Part model, mm, in its own coordinate system. A direction names the side the tool comes from. Round coordinates to 2 decimals unless told otherwise and drop trailing zeros. Loops run counter-clockwise (first coordinate to the right, second up) from the corner with the lowest first, then second, coordinate; pieces in that order, holes last. Notation, with made-up numbers: (12, 43) -> (71, 43) arc R8 ccw to (71, 52) -> close; hole circle Ø2 at (49, 22.25). An arc over 180 degrees is marked (long way). Answer as CSV lines item,"result".
Solid Edge part; units mm, degrees
sketch "Sketch1" plane through (0, 0, 0) normal (0, -1, 0) x (1, 0, 0)
  line L0 (0, 0) -> (22.5, 0)
  line L1 (22.5, 0) -> (22.5, 5)
  line L2 (22.5, 5) -> (-5, 5)
  line L3 (-5, 5) -> (-5, -41)
  line L4 (-5, -41) -> (22.5, -41)
  line L5 (22.5, -41) -> (22.5, -36)
  line L6 (22.5, -36) -> (0, -36)
  line L7 (0, -36) -> (0, 0)
  dimension "D1" = 22.5
  dimension "D2" = 22.5
  dimension "D3" = 22.5
extrude "Protrusion1" add sketch "Sketch1" along normal mid plane 25
sketch "Sketch2" plane through (7.5, 0, 5) normal (0, 0, 1) x (0, 1, 0)
  line L0 (-12.5, 0) -> (-5, -15)
  line L1 (-5, -15) -> (5, -15)
  line L2 (5, -15) -> (12.5, 0)
  line L3 (12.5, 0) -> (12.5, -17.5)
  line L4 (12.5, -17.5) -> (-12.5, -17.5)
  line L5 (-12.5, -17.5) -> (-12.5, 0)
  dimension "D1" = 12.5
  dimension "D2" = 5
extrude "Cutout1" cut sketch "Sketch2" against normal through all
fillet "Round_2" radius 7.5 4 edges at (22.5, -5, 2.5) (22.5, 5, 2.5) (22.5, -5, -38.5) (22.5, 5, -38.5)
hole "Hole_2" at (16, 0, 5) direction (0, 0, -1) diameter 4.5 end through all start chamfer 0.4 start chamfer angle 45 end chamfer 0.4 end chamfer angle 45
hole "Hole_3" at (16, 0, 5) direction (0, 0, -1) diameter 7.2 end up to next
sketch "Sketch3" plane through (7.5, 0, 5) normal (0, 0, 1) x (0, 1, 0)
  line L0 (-3.6, -8.5) -> (3.6, -8.5)
  line L1 (3.6, -8.5) -> (2.4993, 11.5)
  line L2 (2.4993, 11.5) -> (-2.4993, 11.5)
  line L3 (-2.4993, 11.5) -> (-3.6, -8.5)
extrude "ExtrudedCutout_2" cut sketch "Sketch3" against normal blind 2.5
hole "Hole1" at (0, 0, -25.5) direction (-1, 0, 0) diameter 4.5 depth 30 tip angle 118 start chamfer 0.4 start chamfer angle 45 end chamfer 0.4 end chamfer angle 45
hole "Hole2" at (0, 0, -10.5) direction (-1, 0, 0) diameter 4.5 depth 30 tip angle 118 start chamfer 0.4 start chamfer angle 45 end chamfer 0.4 end chamfer angle 45
hole "Hole_8" at (0, -7.5, -18) direction (-1, 0, 0) diameter 3.7 depth 30 tip angle 118 start chamfer 0.6 start chamfer angle 45 end chamfer 0.6 end chamfer angle 45
hole "Hole3" at (0, 7.5, -18) direction (-1, 0, 0) diameter 3.7 depth 30 tip angle 118 start chamfer 0.6 start chamfer angle 45 end chamfer 0.6 end chamfer angle 45
properties material "Polypropylene, general purpose"
Q1. Drop flat-ended pins along their axis: P1, Ø7, axis at x = 16, y = 0, coming from the +Z side; P2, Ø2, axis at y = -8.5, z = 0, coming from the +X side; P3, Ø2, axis at x = 6.5, y = 1.5, coming from the +Z side. Give the stop position or say it passes through.
Geometry results:
P1,"z = -36"
P2,"x = 17.5"
P3,"z = 2.5"
Q2. Saw through at D-D, the plane x = 14.25. Give the number of separate pieces and of enclosed holes in the cut face, then the cut area to 3 significant figures.
Geometry results:
separate pieces,"4"
enclosed holes,"0"
area,"135 mm2"
Q3. Saw through at C-C, the plane x = 3.5. Write the cut outline in (y, z).
Geometry results:
outline,"(-12.5, -41) -> (12.5, -41) -> (12.5, -36) -> (-12.5, -36) -> close; (-12.5, 0) -> (12.5, 0) -> (12.5, 5) -> (2.91, 5) -> (2.91, 2.5) -> (-2.91, 2.5) -> (-2.91, 5) -> (-12.5, 5) -> close"
Q4. Two-plate mould, pull along Z, no slides. Class faces 1 (the face through (-2.529, -0.676, -27.646)), 2 (the face through (21.349, 4.357, 2.465)), 3 (the face through (6, 0, -41)): pulls with the +Z half, pulls with the -Z half, needs draft (parallel to the pull), parting line crosses it, or undercut.
Geometry results:
face 1,"undercut"
face 2,"needs draft"
face 3,"pulls with the -Z half"
Q5. Drill centre lines: line 1 along Z through (x, y) = (-3.65, 0); line 2 along Y through (x, z) = (-2.15, -18); line 3 along X through (y, z) = (0, 2.6). Where is each one in solid material? Low to high.
Geometry results:
line 1,"-41 to -27.75, -23.25 to -12.75, -8.25 to 2.5"
line 2,"-12.5 to -9.35, -5.65 to 5.65, 9.35 to 12.5"
line 3,"-5 to -4, 19.6 to 22.5"
Q6. Which spindle directions (+Z, -Z, +X, -X, +Y, -Y) get a long thin tool onto all of the face, cutting with end or side? Do faces 4 (the face through (13, 9.75, -38.47)), 5 (the face through (0, 0, -18)), 6 (the face through (6, 0, 2.5)). Say none if no direction does.
Geometry results:
face 4,"+Z, -Z, +X, +Y"
face 5,"+X, +Y, -Y"
face 6,"+Z"
Q7. Saw through at A-A, the plane z = -18. Write the cut outline in (x, y), then the cut area to 3 significant figures.
Geometry results:
outline,"(-5, -12.5) -> (0, -12.5) -> (0, -9.95) -> (-0.6, -9.35) -> (-4.4, -9.35) -> (-5, -9.95) -> close; (-5, -5.05) -> (-4.4, -5.65) -> (-0.6, -5.65) -> (0, -5.05) -> (0, 5.05) -> (-0.6, 5.65) -> (-4.4, 5.65) -> (-5, 5.05) -> close; (-5, 9.95) -> (-4.4, 9.35) -> (-0.6, 9.35) -> (0, 9.95) -> (0, 12.5) -> (-5, 12.5) -> close"
area,"86.6 mm2"
Q8. Saw through at B-B, the plane z = -10.5. Write the cut outline in (x, y).
Geometry results:
outline,"(-5, -12.5) -> (0, -12.5) -> (0, -2.65) -> (-0.4, -2.25) -> (-4.6, -2.25) -> (-5, -2.65) -> close; (-5, 2.65) -> (-4.6, 2.25) -> (-0.4, 2.25) -> (0, 2.65) -> (0, 12.5) -> (-5, 12.5) -> close"
